Geometry: final body of the model. Coordinates: model frame, mm. A direction names the side the tool comes from. Give positions to 0.01 mm unless a question says otherwise; leave off trailing zeros. Write each loop counter-clockwise with the first axis right and the second up, starting at its lowest first coordinate (ties: lowest second). Pieces come first, ordered by that corner, then holes. Notation, with made-up numbers: (39.5, -36) -> (87.5, -36) arc R25 cw to (87.5, -8) -> close; hole circle Ø2 at (78.25, 3). An arc over 180 degrees is marked (long way). Answer in a Markdown table with one row per item. Add a question column.
Item 1: First-contact query: P1, Ø4, axis at x = 28.5, y = 5, coming from the -Z side; P2, Ø12, axis at x = 13.5, z = -9.5, coming from the +Y side; P3, Ø2.5, axis at y = 5.5, z = -5, coming from the -X side. Flat tips, straight axial feed; report the tip coordinate or a pass-through.
Item 2: Section query D-D on y = 6. Output: boundary loops of the cut face in (x, z).
Item 3: Section query C-C on x = 7. Output: boundary loops of the cut face in (y, z).
Item 4: Section query B-B on z = -7. Output: boundary loops of the cut face in (x, y).
Item 5: Draft query along X for faces 5 (the flat face through (0, 1, -11)), 6 (the cylindrical face through (27.29, 1.29, -19.88)), 7 (the flat face through (15, 2.54, -11)). Return one class per face: +X half, -X half, draft (parallel to the pull), parting line (faces both ways), or undercut.
Item 6: Access query for faces 1 (the flat face through (22.669, 5, -4)), 2 (the flat face through (27, 5, -1.176)), 3 (the flat face through (30.48, 2, -8)), 4 (the flat face through (27, 5, -7.32)). Directions: +Z, -Z, +X, -X, +Y, -Y. A direction counts if a zero-diameter tool reaches every point of the face in a straight line with its end or side. Return the directions, or none.
Item 7: Section query A-A on z = -2. Output: boundary loops of the cut face in (x, y), plus the area to 3 significant figures.
Item 8: Material intervals for probe 1 along Y at (x, z) = (17.5, -10); probe 2 along Z at (x, y) = (28, 0.5); probe 3 along Z at (x, y) = (14, 2.5), sorted ascending. Write a range as from..to.
```python
from build123d import *

# Parameters (mm, degrees)
SKETCH1_W           = 30.48
SKETCH1_H           = 21.59
BOSS_EXTRUDE1_DEPTH = 2.54
SKETCH2_R           = 1.0922
CUT_EXTRUDE1_DEPTH  = 38.438083551
SKETCH4_W           = 7.811008033
SKETCH4_H           = 6.144185349
BOSS_EXTRUDE2_DEPTH = 5


with BuildPart() as part:
    # Sketch1 → Boss-Extrude1 (new body)
    with BuildSketch(Plane(origin=(0, 0, 0), x_dir=(1, 0, 0), z_dir=(0, 1, 0))):
        with Locations((15.24, 10.795)):
            Rectangle(SKETCH1_W, SKETCH1_H)
    extrude(amount=BOSS_EXTRUDE1_DEPTH)

    # Sketch2 → Cut-Extrude1 (cut, through all)
    with BuildSketch(Plane(origin=(0, 2.54, 0), x_dir=(1, 0, 0), z_dir=(0, 1, 0))):
        with Locations(Location((27.950511617, 19.012165286, 0), (0, 0, 270))):
            Circle(SKETCH2_R)
        with Locations(Location((13.345511617, 2.502165286, 0), (0, 0, 270))):
            Circle(SKETCH2_R)
    extrude(amount=-CUT_EXTRUDE1_DEPTH, mode=Mode.SUBTRACT)

    # Sketch4 → Boss-Extrude2 (add)
    with BuildSketch(Plane(origin=(0, 2.54, 0), x_dir=(1, 0, 0), z_dir=(0, 1, 0))):
        with Locations((26.574495984, 4.247718085)):
            Rectangle(SKETCH4_W, SKETCH4_H)
    extrude(amount=BOSS_EXTRUDE2_DEPTH)


solid = part.part
```
Findings below:
| question | item | result |
|---|---|---|
| 1 | P1 | stops at z = -7.32 |
| 1 | P2 | stops at y = 2.54 |
| 1 | P3 | stops at x = 22.67 |
| 2 | outline | (22.67, -7.32) -> (30.48, -7.32) -> (30.48, -1.18) -> (22.67, -1.18) -> close |
| 3 | outline | (0, -21.59) -> (2.54, -21.59) -> (2.54, 0) -> (0, 0) -> close |
| 4 | outline | (0, 0) -> (30.48, 0) -> (30.48, 7.54) -> (22.67, 7.54) -> (22.67, 2.54) -> (0, 2.54) -> close |
| 5 | face 5 | -X half |
| 5 | face 6 | undercut |
| 5 | face 7 | draft |
| 6 | face 1 | +Z, -Z, -X, +Y |
| 6 | face 2 | +Z, +X, -X, +Y |
| 6 | face 3 | +Z, -Z, +X, +Y, -Y |
| 6 | face 4 | -Z, +X, -X, +Y |
| 7 | outline | (0, 0) -> (12.38, 0) -> (12.38, 2.54) -> (0, 2.54) -> close; (14.32, 0) -> (30.48, 0) -> (30.48, 7.54) -> (22.67, 7.54) -> (22.67, 2.54) -> (14.32, 2.54) -> close |
| 7 | area | 112 mm^2 |
| 8 | probe 1 | y = 0..2.54 |
| 8 | probe 2 | z = -21.59..-20.1, -17.92..0 |
| 8 | probe 3 | z = -21.59..-3.38, -1.63..0 |
